Geometry check sheet. Reference: the model listing, model coordinates, mm. A direction names the side the tool comes from. Round coordinates to 2 decimals unless told otherwise and drop trailing zeros. Order: outer loops, then holes, each group sorted by start corner. A loop starts at its lowest first (then second) coordinate and runs counter-clockwise, first axis right, second up.
```python
from build123d import *

# Parameters (mm, degrees)
SKETCH1_R           = 11.557
SKETCH1_R_2         = 2.6
SKETCH1_R_3         = 2.4
BOSS_EXTRUDE1_DEPTH = 10
BOSS_EXTRUDE2_DEPTH = 16


with BuildPart() as part:
    # Sketch1 → Boss-Extrude1 (new body)
    with BuildSketch(Plane(origin=(0, 0, 0), x_dir=(0, 0, -1), z_dir=(1, 0, 0))):
        Circle(SKETCH1_R)
        with Locations((8, 0)):
            Circle(SKETCH1_R_2, mode=Mode.SUBTRACT)
        with Locations((0, -8)):
            Circle(SKETCH1_R_2, mode=Mode.SUBTRACT)
        with Locations((-8, 0)):
            Circle(SKETCH1_R_2, mode=Mode.SUBTRACT)
        with Locations((0, 8)):
            Circle(SKETCH1_R_3, mode=Mode.SUBTRACT)
    extrude(amount=BOSS_EXTRUDE1_DEPTH)

    # Sketch2 → Boss-Extrude2 (add)
    with BuildSketch(Plane(origin=(10, 0, 0), x_dir=(0, 0, -1), z_dir=(1, 0, 0))):
        with BuildLine():
            Line((1.25, 2.165063509), (-1.25, 2.165063509))
            ThreePointArc((-1.25, 2.165063509), (-1.25, -2.165063509), (2.5, 0))
            ThreePointArc((2.5, 0), (2.165063509, 1.25), (1.25, 2.165063509))
        make_face()
    extrude(amount=BOSS_EXTRUDE2_DEPTH)


solid = part.part
```
(1) Depth check by flat-ended pin: P1, Ø3, axis at x = 16, y = 1.5, coming from the +Z side; P2, Ø2, axis at y = 6, z = -2.5, coming from the +X side; P3, Ø1, axis at x = 6.5, z = -3, coming from the +Y side; P4, Ø4.5, axis at y = 0, z = 8, coming from the +X side. Enter the tip coordinate at first touch or a pass-through.
Returned:
P1: stops at z = 2.5
P2: stops at x = 10
P3: stops at y = 11.28
P4: passes through
(2) Sectioned sample at B-B, the plane y = -8. Record the cut outline in (x, z), and give its area (3 significant figures).
Returned:
outline: (0, -8.34) - (10, -8.34) - (10, -2.6) - (0, -2.6) - close; (0, 2.6) - (10, 2.6) - (10, 8.34) - (0, 8.34) - close
area: 115 mm2
(3) Sectioned sample at C-C, the plane z = 0. Record the cut outline in (x, y).
Returned:
outline: (0, -11.56) - (10, -11.56) - (10, -10.6) - (0, -10.6) - close; (0, -5.4) - (10, -5.4) - (10, -2.5) - (26, -2.5) - (26, 2.17) - (10, 2.17) - (10, 5.6) - (0, 5.6) - close; (0, 10.4) - (10, 10.4) - (10, 11.56) - (0, 11.56) - close
(4) Material ranges on line 1 (Y direction, x = 8.25, z = 0); line 2 (X direction, y = 6, z = -6); line 3 (Z direction, x = 4.5, y = -1), recorded low to high.
Returned:
line 1: y = -11.56 to -10.6, -5.4 to 5.6, 10.4 to 11.56
line 2: x = 0 to 10
line 3: z = -11.51 to -10.4, -5.6 to 5.6, 10.4 to 11.51
(5) Set-up check for faces 4 (the cylindrical face through (4.93, 0.78, -10.48)), 5 (the flat face through (18, 2.165, 0)): record each of +Z, -Z, +X, -X, +Y, -Y from which the full face is reachable in a straight line by a thin tool's end or side.
Returned:
face 4: +X, -X
face 5: +Z, -Z, +X, +Y
(6) Sectioned sample at D-D, the plane x = 7.5. Record the cut outline in (y, z).
Returned:
outline: circle Ø23.11 at (0, 0); hole circle Ø5.2 at (-8, 0); hole circle Ø5.2 at (0, -8); hole circle Ø5.2 at (0, 8); hole circle Ø4.8 at (8, 0)
(7) Sectioned sample at A-A, the plane z = -10. Record the cut outline in (x, y), and give its area (3 significant figures).
Returned:
outline: (0, -5.79) - (10, -5.79) - (10, -1.66) - (0, -1.66) - close; (0, 1.66) - (10, 1.66) - (10, 5.79) - (0, 5.79) - close
area: 82.6 mm2
(8) Draft check along Z on faces 1 (the flat face through (10, 3, 0)), 2 (the cylindrical face through (4.93, 9.745, -6.213)), 3 (the cylindrical face through (4.93, 2.578, 8.338)). Enter one of: released by +Z, released by -Z, zero draft, split by the parting line, or undercut.
Returned:
face 1: zero draft
face 2: split by the parting line
face 3: undercut
